```python
from build123d import *

# Parameters (mm, degrees)
CROQUIS1_W              = 37.6
CROQUIS1_H              = 6.1
SALIENTE_EXTRUIR1_DEPTH = 8.9
CROQUIS2_W              = 35.8
CROQUIS2_H              = 4.3
CROQUIS2_W_2            = 15
CROQUIS2_H_2            = 0.9
CORTAR_EXTRUIR2_DEPTH   = 8.9
CROQUIS3_W              = 5.5
CROQUIS3_H              = 3.9
CORTAR_EXTRUIR3_DEPTH   = 8.9
REDONDEO1_R             = 2
REDONDEO2_START         = 5.2
REDONDEO2_DEPTH         = 0.9
REDONDEO2_2_DEPTH       = 0.9
REDONDEO4_R             = 1
REDONDEO5_R             = 1
REDONDEO6_R             = 1
REDONDEO7_R             = 1
REDONDEO8_R             = 1
REDONDEO9_R             = 1
REDONDEO10_R            = 1
REDONDEO11_R            = 1
REDONDEO12_R            = 1
REDONDEO13_R            = 1
REDONDEO14_R            = 1
REDONDEO15_R            = 1


with BuildPart() as part:
    # Croquis1 → Saliente-Extruir1 (new body)
    with BuildSketch(Plane.XY):
        with Locations((18.8, 3.05)):
            Rectangle(CROQUIS1_W, CROQUIS1_H)
    extrude(amount=SALIENTE_EXTRUIR1_DEPTH)

    # Croquis2 → Cortar-Extruir2 (cut)
    with BuildSketch(Plane.XY.offset(8.9)):
        with Locations((18.8, 3.05)):
            Rectangle(CROQUIS2_W, CROQUIS2_H)
        with Locations((18.8, 5.65)):
            Rectangle(CROQUIS2_W_2, CROQUIS2_H_2)
    extrude(amount=-CORTAR_EXTRUIR2_DEPTH, mode=Mode.SUBTRACT)

    # Croquis3 → Cortar-Extruir3 (cut)
    with BuildSketch(Plane(origin=(0, 0, 0), x_dir=(1, 0, 0), z_dir=(0, 1, 0))):
        with Locations((6.335, -4.45)):
            Rectangle(CROQUIS3_W, CROQUIS3_H)
        with Locations((31.265, -4.45)):
            Rectangle(CROQUIS3_W, CROQUIS3_H)
    extrude(amount=CORTAR_EXTRUIR3_DEPTH, mode=Mode.SUBTRACT)

    # Redondeo1
    redondeo1_edges = [part.edges().sort_by_distance(p)[0] for p in [
        (3.585, 0.45, 6.4),
    ]]
    fillet(redondeo1_edges, radius=REDONDEO1_R)


with BuildPart() as redondeo2_tool:
    # Redondeo2: read off the stored shape, not the designer's step
    # Redondeo2 outline → Redondeo2 (new body)
    with BuildSketch(Plane(origin=(0, 0, 0), x_dir=(1, 0, 0), z_dir=(0, 1, 0)).offset(REDONDEO2_START)):
        with BuildLine():
            ThreePointArc((5.585, -6.4), (4.188575996, -5.831782106), (3.585625098, -4.45))
            ThreePointArc((3.585625098, -4.45), (4.187680846, -3.069091484), (5.582498438, -2.500001564))
            Line((5.582498438, -2.500001564), (3.585, -2.5))
            Line((3.585, -2.5), (3.585, -6.4))
            Line((3.585, -6.4), (5.585, -6.4))
        make_face()
        with BuildLine():
            ThreePointArc((9.084374902, -4.45), (8.481424004, -5.831782106), (7.085, -6.4))
            Line((7.085, -6.4), (9.085, -6.4))
            Line((9.085, -6.4), (9.085, -2.5))
            Line((9.085, -2.5), (7.085, -2.5))
            ThreePointArc((7.085, -2.5), (8.481424004, -3.068217894), (9.084374902, -4.45))
        make_face()
        with BuildLine():
            ThreePointArc((28.515625098, -4.45), (29.118575996, -3.068217894), (30.515, -2.5))
            Line((30.515, -2.5), (28.515, -2.5))
            Line((28.515, -2.5), (28.515, -6.4))
            Line((28.515, -6.4), (30.515, -6.4))
            ThreePointArc((30.515, -6.4), (29.118575996, -5.831782106), (28.515625098, -4.45))
        make_face()
        with BuildLine():
            Line((34.015, -2.5), (32.015, -2.5))
            ThreePointArc((32.015, -2.5), (33.411424004, -3.068217894), (34.014374902, -4.45))
            ThreePointArc((34.014374902, -4.45), (33.411424004, -5.831782106), (32.015, -6.4))
            Line((32.015, -6.4), (34.015, -6.4))
            Line((34.015, -6.4), (34.015, -2.5))
        make_face()
    extrude(amount=REDONDEO2_DEPTH)


with BuildPart() as part_1:
    add(part.part)


with BuildPart() as part_2:
    # Redondeo2: joined with redondeo2_tool
    add(part_1.part.fuse(redondeo2_tool.part, tol=0.00001))


with BuildPart() as redondeo2_2_tool:
    # Redondeo2 2 outline → Redondeo2 2 (new body)
    with BuildSketch(Plane(origin=(0, 0, 0), x_dir=(1, 0, 0), z_dir=(0, 1, 0))):
        with BuildLine():
            ThreePointArc((3.585, -4.4), (4.20409356, -3.050862325), (5.582498436, -2.5))
            Line((5.582498436, -2.5), (3.585, -2.5))
            Line((3.585, -2.5), (3.585, -4.4))
        make_face()
        with BuildLine():
            ThreePointArc((9.084374902, -4.45), (8.481424004, -5.831782106), (7.085, -6.4))
            Line((7.085, -6.4), (9.085, -6.4))
            Line((9.085, -6.4), (9.085, -2.5))
            Line((9.085, -2.5), (7.085, -2.5))
            ThreePointArc((7.085, -2.5), (8.481424004, -3.068217894), (9.084374902, -4.45))
        make_face()
        with BuildLine():
            ThreePointArc((28.515625098, -4.45), (29.118575996, -3.068217894), (30.515, -2.5))
            Line((30.515, -2.5), (28.515, -2.5))
            Line((28.515, -2.5), (28.515, -6.4))
            Line((28.515, -6.4), (30.515, -6.4))
            ThreePointArc((30.515, -6.4), (29.118575996, -5.831782106), (28.515625098, -4.45))
        make_face()
        with BuildLine():
            Line((34.015, -2.5), (32.015, -2.5))
            ThreePointArc((32.015, -2.5), (33.411424004, -3.068217894), (34.014374902, -4.45))
            ThreePointArc((34.014374902, -4.45), (33.411424004, -5.831782106), (32.015, -6.4))
            Line((32.015, -6.4), (34.015, -6.4))
            Line((34.015, -6.4), (34.015, -2.5))
        make_face()
    extrude(amount=REDONDEO2_2_DEPTH)


with BuildPart() as part_3:
    add(part_2.part)


with BuildPart() as part_4:
    # Redondeo2 2: joined with redondeo2_2_tool
    add(part_3.part.fuse(redondeo2_2_tool.part, tol=0.00001))

    # Redondeo4
    redondeo4_edges = [part_4.edges().sort_by_distance(p)[0] for p in [
        (0, 0, 4.45),
    ]]
    fillet(redondeo4_edges, radius=REDONDEO4_R)

    # Redondeo5
    redondeo5_edges = [part_4.edges().sort_by_distance(p)[0] for p in [
        (37.6, 0, 4.45),
    ]]
    fillet(redondeo5_edges, radius=REDONDEO5_R)

    # Redondeo6
    redondeo6_edges = [part_4.edges().sort_by_distance(p)[0] for p in [
        (37.6, 6.1, 4.45),
    ]]
    fillet(redondeo6_edges, radius=REDONDEO6_R)

    # Redondeo7
    redondeo7_edges = [part_4.edges().sort_by_distance(p)[0] for p in [
        (0, 6.1, 4.45),
    ]]
    fillet(redondeo7_edges, radius=REDONDEO7_R)

    # Redondeo8
    redondeo8_edges = [part_4.edges().sort_by_distance(p)[0] for p in [
        (0.9, 0.9, 4.45),
    ]]
    fillet(redondeo8_edges, radius=REDONDEO8_R)

    # Redondeo9
    redondeo9_edges = [part_4.edges().sort_by_distance(p)[0] for p in [
        (0.9, 5.2, 4.45),
    ]]
    fillet(redondeo9_edges, radius=REDONDEO9_R)

    # Redondeo10
    redondeo10_edges = [part_4.edges().sort_by_distance(p)[0] for p in [
        (36.7, 0.9, 4.45),
    ]]
    fillet(redondeo10_edges, radius=REDONDEO10_R)

    # Redondeo11
    redondeo11_edges = [part_4.edges().sort_by_distance(p)[0] for p in [
        (36.7, 5.2, 4.45),
    ]]
    fillet(redondeo11_edges, radius=REDONDEO11_R)

    # Redondeo12
    redondeo12_edges = [part_4.edges().sort_by_distance(p)[0] for p in [
        (26.3, 5.65, 8.9),
    ]]
    fillet(redondeo12_edges, radius=REDONDEO12_R)

    # Redondeo13
    redondeo13_edges = [part_4.edges().sort_by_distance(p)[0] for p in [
        (26.3, 5.65, 0),
    ]]
    fillet(redondeo13_edges, radius=REDONDEO13_R)

    # Redondeo14
    redondeo14_edges = [part_4.edges().sort_by_distance(p)[0] for p in [
        (11.3, 5.65, 0),
    ]]
    fillet(redondeo14_edges, radius=REDONDEO14_R)

    # Redondeo15
    redondeo15_edges = [part_4.edges().sort_by_distance(p)[0] for p in [
        (11.3, 5.65, 8.9),
    ]]
    fillet(redondeo15_edges, radius=REDONDEO15_R)


solid = part_4.part
```
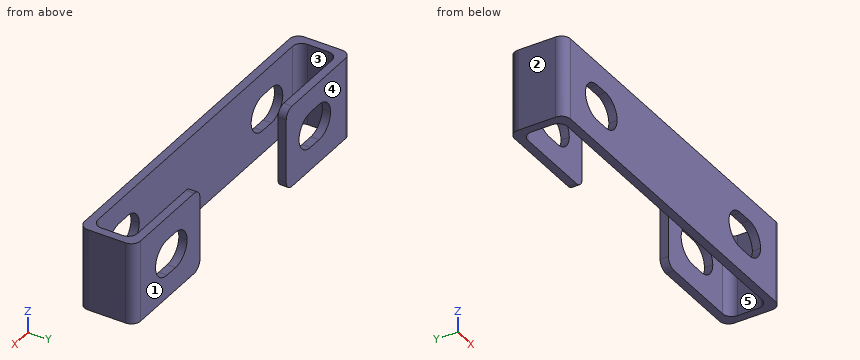
Read the model definition and answer for the solid it produces. Units are mm, in the model's axes. Face numbers are marked on the shaded views. A direction names the side the tool comes from. Give positions to 0.01 mm unless a question says otherwise; leave off trailing zeros. Loops run counter-clockwise (first coordinate to the right, second up) from the corner with the lowest first, then second, coordinate; pieces in that order, holes last.
Item 1: The mould has two halves that part along X. Classify the marked faces 1, 2 and 3: released by +X, released by -X, zero draft, split by the parting line, or undercut.
Item 2: Each of these flat-tipped pins is pushed along its axis until it touches: pin 1 Ø1 at (x, y) = (31, 0.5) entering from -Z; pin 2 Ø0.5 at (y, z) = (5.5, 4.5) entering from -X; pin 3 Ø1 at (x, y) = (11, 5) entering from +Z. Where does it stop, or does it pass through?
Item 3: The part is cut by section A-A (y = 2.75). Write down the section's boundary in (x, z).
Item 4: Find the intervals of material crossed by line 1 along X through (y, z) = (3, 0.5); line 2 along Y through (x, z) = (11, 0.75); line 3 along Y through (x, z) = (26, 6), in increasing order.
Item 5: For the marked faces 4 and 5, determine the directions among +Z, -Z, +X, -X, +Y, -Y from which every point of the face is accessible in a straight line to the end or side of a thin tool.
Item 6: The part is cut by section B-B (x = 35). Write down the section's boundary in (y, z), and give its area (3 significant figures).
Item 7: The part is cut by section C-C (y = 5.75). Give the number of separate pieces and of enclosed holes in the cut face, and give its area (3 significant figures).
Item 8: The part is cut by section D-D (z = 2). Write down the section's boundary in (x, y), and give its area (3 significant figures).
Taken from the geometry:
1. face 1: zero draft
1. face 2: released by -X
1. face 3: undercut
2. pin 1: stops at z = 0
2. pin 2: stops at x = 0.01
2. pin 3: stops at z = 8.87
3. outline: (0, 0) - (0.9, 0) - (0.9, 8.9) - (0, 8.9) - close; (36.7, 0) - (37.6, 0) - (37.6, 8.9) - (36.7, 8.9) - close
4. line 1: x = 0 to 0.9, 36.7 to 37.6
4. line 2: y = 0 to 0.9, 5.2 to 6.1
4. line 3: y = 0 to 0.9
5. face 4: +Z, -Z, +X, -X, +Y
5. face 5: +Z, -Z
6. outline: (0, 0) - (0.9, 0) - (0.9, 8.9) - (0, 8.9) - close; (5.2, 0) - (6.1, 0) - (6.1, 8.9) - (5.2, 8.9) - close
6. area: 16.0 mm2
7. separate pieces: 2
7. enclosed holes: 2
7. area: 160 mm2
8. outline: (0, 1) arc R1 ccw to (1, 0) - (36.6, 0) arc R1 ccw to (37.6, 1) - (37.6, 5.1) arc R1 ccw to (36.6, 6.1) - (26.3, 6.1) - (26.3, 5.2) - (35.7, 5.2) arc R1 cw to (36.7, 4.2) - (36.7, 1.9) arc R1 cw to (35.7, 0.9) - (1.9, 0.9) arc R1 cw to (0.9, 1.9) - (0.9, 4.2) arc R1 cw to (1.9, 5.2) - (11.3, 5.2) - (11.3, 6.1) - (1, 6.1) arc R1 ccw to (0, 5.1) - close
8. area: 61.9 mm2
